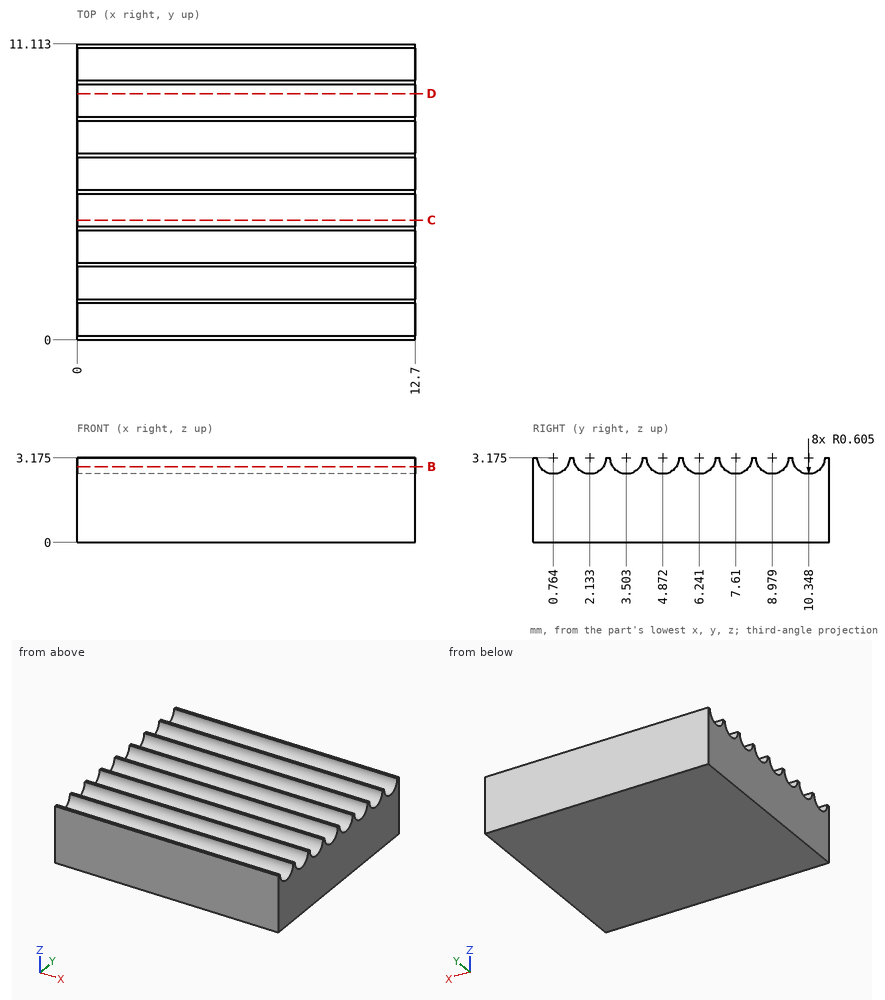
Geometry: see drawing. Coordinates: mm, zero at the bounding-box minimum. Round coordinates to 2 decimals unless told otherwise and drop trailing zeros. Write each loop counter-clockwise with the first axis right and the second up, starting at its lowest first coordinate (ties: lowest second). Pieces come first, ordered by that corner, then holes. Notation, with made-up numbers: M 12,44 L 40,44 A20 cw 40,61 Z; hole C 29,64.5 d11. An arc over 180 degrees is marked long. Answer as a JSON object with one key per item and string values. Group by question number.
(1) Ray query, line 1 (Z direction, x = 6, y = 3.5); line 2 (Z direction, x = 8.75, y = 4) (1 decimal). Return the intervals inside material, ascending. Write a range as [from, to].
(2) Section query C-C on y = 4.5. Output: boundary loops of the cut face in (x, z).
(3) Section query D-D on y = 9.25. Output: boundary loops of the cut face in (x, z) (1 decimal).
(4) Section query B-B on z = 2.85. State how many separate pieces and enclosed holes the cut face has.
Computed values:
{
 "1": {"line 1": "[0, 2.57]", "line 2": "[0, 2.8]"},
 "2": {"outline": "M 0,0 L 12.7,0 L 12.7,2.7 L 0,2.7 Z"},
 "3": {"outline": "M 0,0 L 12.7,0 L 12.7,2.6 L 0,2.6 Z"},
 "4": {"separate pieces": "9", "enclosed holes": "0"}
}
